Part model, mm, in its own coordinate system. Coordinates: 2 decimals unless noted, no trailing zeros. Loops run counter-clockwise (first coordinate to the right, second up) from the corner with the lowest first, then second, coordinate; pieces in that order, holes last.
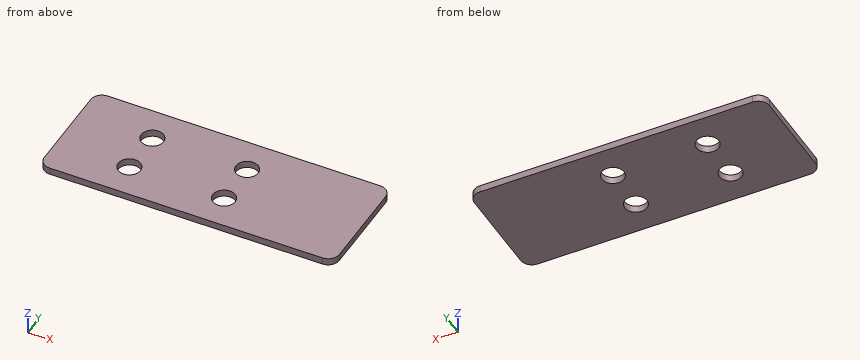
Autodesk Inventor part; units mm, degrees
ref_plane "YZ Plane" through (0, 0, 0) normal (1, 0, 0) x (0, 1, 0)
ref_plane "XZ Plane" through (0, 0, 0) normal (0, 1, 0) x (-1, 0, 0)
ref_plane "XY Plane" through (0, 0, 0) normal (0, 0, 1) x (1, 0, 0)
sketch "Base" plane through (0, 0, 0) normal (0, 0, 1) x (1, 0, 0)
  line L0 (0, 0) -> (12.7, 0) construction
  line L1 (12.7, -15.9583) -> (-70.993, -15.9583) construction
  line L2 (12.7, 0) -> (12.7, -15.9583) construction
  line L3 (12.7, -31.9166) -> (12.7, -15.9583) construction
  line L4 (0, -31.9166) -> (12.7, -31.9166) construction
  circle A0 centre (-23.3035, -22.3083) radius 3.175
  circle A1 centre (-50.1821, -22.3083) radius 3.175
  circle A2 centre (-50.1821, -22.3083) radius 3.175
  circle A3 centre (-23.3035, -9.6083) radius 3.175
  circle A4 centre (-50.1821, -9.6083) radius 3.175
  line L5 (-50.1821, -9.6083) -> (-23.3035, -9.6083) construction
  line L6 (-50.1821, -22.3083) -> (-23.3035, -22.3083) construction
  line L7 (-50.1821, -9.6083) -> (-50.1821, -22.3083) construction
  line L8 (-23.3035, -9.6083) -> (-23.3035, -22.3083) construction
  line L9 (0, 0) -> (-70.993, 0) construction
  line L10 (0, -31.9166) -> (-70.993, -31.9166) construction
  line L11 (-70.993, -31.9166) -> (-70.993, 0) construction
  line L12 (-70.993, 0) -> (12.7, 0)
  line L13 (12.7, 0) -> (12.7, -31.9166)
  line L14 (12.7, -31.9166) -> (-70.993, -31.9166)
  line L15 (-70.993, -31.9166) -> (-70.993, 0)
  dimension "d0" = 6.35
  dimension "d1" = 6.35
  dimension "d2" = 180
  dimension "d3" = 90
  dimension "d4" = 36.0035
  dimension "d5" = 62.8821
  dimension "d6" = 83.693
  dimension "d7" = 15.9583
  dimension "d8" = 6.35
  dimension "d9" = 6.35
  dimension "d10" = 12.7
  dimension "d11" = 12.7
  dimension "d12" = 15.9583
  dimension "d13" = 0
  dimension "d14" = 12.7
  dimension "d15" = 12.7
  dimension "d16" = 62.8821
  dimension "d17" = 6.35
extrude "Plate1" add sketch "Base" along normal blind 2
fillet "Corner Round1" radius 3.175 4 edges at (12.7, -31.9166, 1) (12.7, 0, 1) (-70.993, -31.9166, 1) (-70.993, 0, 1)
equation "\"d18\" = Thickness"
equation "\"BendRadius\" = Thickness"
equation "\"BendReliefWidth\" = Thickness"
equation "\"BendReliefDepth\" = 0.5 * Thickness"
equation "\"CornerReliefSize\" = 4 * Thickness"
equation "\"MinimumRemnant\" = 2 * Thickness"
equation "\"TransitionRadius\" = BendRadius"
equation "\"JacobiRadiusSize\" = BendRadius"
equation "\"GapSize\" = Thickness"
properties part number "StockMountPlate"
Q1. Saw through at C-C (z = 0.4). Count the separate pieces of the cut face and the enclosed holes in it, plus the area to 3 significant figures.
Q2. Saw through at B-B (x = -51). List the corners of the cut face in (y, z).
Q3. Probe line 1 (X direction, y = -22, z = 1.7); line 2 (X direction, y = -24.5, z = 0.8); line 3 (Y direction, x = -49.5, z = 0.2). List the from-to ranges inside material, lowest first.
Q4. Saw through at A-A (y = -11.5). List the corners of the cut face in (x, z), plus the area to 3 significant figures.
Checked values:
1. separate pieces: 1
1. enclosed holes: 4
1. area: 2,540 mm2
2. outline: (-31.92, 0) - (-25.38, 0) - (-25.38, 2) - (-31.92, 2) - close; (-19.24, 0) - (-12.68, 0) - (-12.68, 2) - (-19.24, 2) - close; (-6.54, 0) - (0, 0) - (0, 2) - (-6.54, 2) - close
3. line 1: x = -70.99 to -53.34, -47.02 to -26.46, -20.14 to 12.7
3. line 2: x = -70.99 to -52.48, -47.88 to -25.6, -21.01 to 12.7
3. line 3: y = -31.92 to -25.41, -19.21 to -12.71, -6.51 to 0
4. outline: (-70.99, 0) - (-52.73, 0) - (-52.73, 2) - (-70.99, 2) - close; (-47.63, 0) - (-25.85, 0) - (-25.85, 2) - (-47.63, 2) - close; (-20.75, 0) - (12.7, 0) - (12.7, 2) - (-20.75, 2) - close
4. area: 147 mm2
